Autodesk Inventor part; units mm, degrees
ref_plane "YZ Plane" through (0, 0, 0) normal (1, 0, 0) x (0, 1, 0)
ref_plane "XZ Plane" through (0, 0, 0) normal (0, 1, 0) x (-1, 0, 0)
ref_plane "XY Plane" through (0, 0, 0) normal (0, 0, 1) x (1, 0, 0)
sketch "Skizze1" plane through (0, 0, 0) normal (0, 1, 0) x (-1, 0, 0)
  circle A0 centre (0, 0) radius 15
  dimension "d0" = 30
extrude "Extrusion1" add sketch "Skizze1" along normal blind 150
sketch "Skizze2" plane through (0, 150, 0) normal (0, 1, 0) x (1, 0, 0)
  line L0 (-16, -5) -> (-6, -5)
  line L1 (-6, -5) -> (-6, 5)
  line L2 (-6, 5) -> (-16, 5)
  line L3 (-16, 5) -> (-16, -5)
  line L4 (-22.2, 0) -> (21.2, 0) construction
  line L5 (0, 21) -> (0, -21) construction
  dimension "d3" = 6
  dimension "d4" = 10
  dimension "d5" = 10
extrude "Extrusion2" cut sketch "Skizze2" against normal blind 44.6
sketch "Skizze3" plane through (0, 0, 0) normal (0, -1, 0) x (1, 0, 0)
  line L0 (-18, -3) -> (-6, -3)
  line L1 (-6, -3) -> (-6, 3)
  line L2 (-6, 3) -> (-18, 3)
  line L3 (-18, 3) -> (-18, -3)
  line L4 (-24.6, 0) -> (21.6, 0) construction
  line L5 (0, -21) -> (0, 21) construction
  dimension "d8" = 6
  dimension "d9" = 12
  dimension "d10" = 6
extrude "Extrusion3" cut sketch "Skizze3" against normal blind 20
properties part number "Welle_000"
Read the model definition and answer for the solid it produces. Units are mm, in the model's axes. A direction names the side the tool comes from. Give positions to 0.01 mm unless a question says otherwise; leave off trailing zeros. Write each loop counter-clockwise with the first axis right and the second up, starting at its lowest first coordinate (ties: lowest second). Pieces come first, ordered by that corner, then holes. Notation, with made-up numbers: (-1.5, -36) -> (30.5, -36) arc R19 cw to (30.5, -14) -> close; hole circle Ø7 at (77.25, -19). An arc over 180 degrees is marked (long way). Answer in a Markdown table with one row per item.
1) Section D-D on y = 9 is taken. Give the vertices of the cut face in (x, z).
Results list:
| item | result |
|---|---|
| outline | (-14.7, -3) arc R15 ccw (long way) to (-14.7, 3) -> (-6, 3) -> (-6, -3) -> close |
2) Determine the mould class of faces 1 (the flat face through (0, 0, 0)), 2 (the cylindrical face through (14.985, 73.95, -0.66)), 3 (the flat face through (-10, 128, 5)) for opening direction Z: released by +Z, released by -Z, zero draft, split by the parting line, or undercut.
Results list:
| item | result |
|---|---|
| face 1 | zero draft |
| face 2 | split by the parting line |
| face 3 | undercut |
3) Section A-A on z = 0 is taken. Give the vertices of the cut face in (x, y).
Results list:
| item | result |
|---|---|
| outline | (-15, 20) -> (-6, 20) -> (-6, 0) -> (15, 0) -> (15, 150) -> (-6, 150) -> (-6, 105.4) -> (-15, 105.4) -> close |
4) Section C-C on y = 78.5 is taken. Give the vertices of the cut face in (x, z), plus the area to 3 significant figures.
Results list:
| item | result |
|---|---|
| outline | circle Ø30 at (0, 0) |
| area | 707 mm^2 |
5) Section B-B on x = -11.75 is taken. Give the vertices of the cut face in (y, z), plus the area to 3 significant figures.
Results list:
| item | result |
|---|---|
| outline | (0, -9.32) -> (150, -9.32) -> (150, -5) -> (105.4, -5) -> (105.4, 5) -> (150, 5) -> (150, 9.32) -> (0, 9.32) -> (0, 3) -> (20, 3) -> (20, -3) -> (0, -3) -> close |
| area | 2,230 mm^2 |
6) A tool of negligible diameter and unlimited length cuts with its end or side. For faces 4 (the flat face through (1, 150, 0)), 5 (the flat face through (-10, 10, 3)), 6 (the flat face through (-11, 105.4, 0)), from which of +Z, -Z, +X, -X, +Y, -Y can it reach the whole face along a straight path? Write none if from no direction.
Results list:
| item | result |
|---|---|
| face 4 | +Z, -Z, +X, -X, +Y |
| face 5 | -X, -Y |
| face 6 | -X, +Y |
7) Each of these flat-tipped pins is pushed along its axis until it touches: pin 1 Ø12 at (y, z) = (34, 10) entering from -X; pin 2 Ø4 at (y, z) = (72, 3.5) entering from +X; pin 3 Ø6.5 at (y, z) = (8.5, 0) entering from -X. Where does it stop, or does it pass through?
Results list:
| item | result |
|---|---|
| pin 1 | x = -14.46 |
| pin 2 | x = 14.92 |
| pin 3 | x = -14.7 |
8) Straight lines are drawn through the part: line 1 (Y direction, x = -11.75, z = 4.5); line 2 (Z direction, x = -9, y = 105.5); line 3 (Z direction, x = -9.5, y = 105.5). For each, find the intervals that lie inside material, in ascending order. Write a range as [from, to].
Results list:
| item | result |
|---|---|
| line 1 | [0, 105.4] |
| line 2 | [-12, -5], [5, 12] |
| line 3 | [-11.61, -5], [5, 11.61] |
